Geometry check sheet. Reference: the model listing, model coordinates, mm. A direction names the side the tool comes from. Round coordinates to 2 decimals unless told otherwise and drop trailing zeros. Order: outer loops, then holes, each group sorted by start corner. A loop starts at its lowest first (then second) coordinate and runs counter-clockwise, first axis right, second up.
Autodesk Inventor part; units mm, degrees
ref_plane "Work Plane1" through (0, 0, 0) normal (0, 0, 1) x (1, 0, 0)
ref_plane "Work Plane2" through (0.04, -9.12, 0) normal (1, 0, 0) x (0, 0, -1)
ref_plane "YZ Plane" through (0, 0, 0) normal (1, 0, 0) x (0, 1, 0)
ref_plane "Work Plane1" through (0, 0, 0) normal (0, 0, 1) x (1, 0, 0)
sketch "Sketch1" plane through (0, 0, 0) normal (0, 0, 1) x (1, 0, 0)
  circle A0 centre (2.54, -6.27) radius 0.302
  circle A1 centre (-2.46, -6.27) radius 0.302
  line L0 (2.54, -6.27) -> (-2.46, -6.27)
  line L1 (2.89, -9.37) -> (-2.81, -9.37)
  line L2 (-3.06, -9.12) -> (-3.06, -3.42)
  line L3 (-2.81, -3.17) -> (2.89, -3.17)
  line L4 (3.14, -3.42) -> (3.14, -9.12)
  line L5 (3.14, -9.37) -> (-3.06, -3.17) construction
  line L6 (-3.06, -9.37) -> (3.14, -3.17) construction
  arc A2 (2.89, -9.37) -> (3.14, -9.12) centre (2.89, -9.12) ccw
  arc A3 (-3.06, -9.12) -> (-2.81, -9.37) centre (-2.81, -9.12) ccw
  arc A4 (-2.81, -3.17) -> (-3.06, -3.42) centre (-2.81, -3.42) ccw
  arc A5 (3.14, -3.42) -> (2.89, -3.17) centre (2.89, -3.42) ccw
  point P0 (0, 0)
  point P1 (0.04, -6.27)
  dimension "d0" = 6.2
  dimension "d1" = 6.2
  dimension "d2" = 0.25
extrude "Extrusion1" add sketch "Sketch1" along normal blind 3.4 contours A0 | A1 | L1 A3 L2 A4 L3 A5 L4 A2
sketch "Sketch2" plane through (0, 0, 3.4) normal (0, 0, 1) x (1, 0, 0)
  arc A0 (2.89, -9.37) -> (3.14, -9.12) centre (2.89, -9.12) ccw
  line L0 (3.14, -9.12) -> (3.14, -3.42)
  arc A1 (3.14, -3.42) -> (2.89, -3.17) centre (2.89, -3.42) ccw
  line L1 (2.89, -3.17) -> (-2.81, -3.17)
  arc A2 (-2.81, -3.17) -> (-3.06, -3.42) centre (-2.81, -3.42) ccw
  line L2 (-3.06, -3.42) -> (-3.06, -9.12)
  arc A3 (-3.06, -9.12) -> (-2.81, -9.37) centre (-2.81, -9.12) ccw
  line L3 (-2.81, -9.37) -> (2.89, -9.37)
  line L4 (-1.885, -4.345) -> (1.965, -8.195) construction
  line L5 (1.965, -4.345) -> (-1.885, -8.195) construction
  circle A4 centre (1.965, -4.345) radius 0.45
  circle A5 centre (1.965, -8.195) radius 0.45
  circle A6 centre (-1.885, -8.195) radius 0.45
  circle A7 centre (-1.885, -4.345) radius 0.45
  point P0 (0, 0)
  point P1 (0.04, -6.27)
  dimension "d5" = 3.85
  dimension "d6" = 3.85
  dimension "d7" = 0.9
  dimension "d8" = 0.9
  dimension "d9" = 0.9
  dimension "d10" = 0.9
extrude "Extrusion2" add sketch "Sketch2" along normal blind 0.4 contours A4 | A5 | A6 | A7
fillet "Fillet1" radius 0.1 4 edges at (1.515, -4.345, 3.8) (1.515, -8.195, 3.8) (-2.335, -8.195, 3.8) (-2.335, -4.345, 3.8)
sketch "Sketch3" plane through (0, 0, 3.4) normal (0, 0, 1) x (1, 0, 0)
  circle A0 centre (-1.885, -8.195) radius 0.45
  circle A1 centre (1.965, -8.195) radius 0.45
  circle A2 centre (-1.885, -4.345) radius 0.45
  circle A3 centre (1.965, -4.345) radius 0.45
  arc A4 (2.89, -9.37) -> (3.14, -9.12) centre (2.89, -9.12) ccw
  line L0 (3.14, -9.12) -> (3.14, -3.42)
  arc A5 (3.14, -3.42) -> (2.89, -3.17) centre (2.89, -3.42) ccw
  line L1 (2.89, -3.17) -> (-2.81, -3.17)
  arc A6 (-2.81, -3.17) -> (-3.06, -3.42) centre (-2.81, -3.42) ccw
  line L2 (-3.06, -3.42) -> (-3.06, -9.12)
  arc A7 (-3.06, -9.12) -> (-2.81, -9.37) centre (-2.81, -9.12) ccw
  line L3 (-2.81, -9.37) -> (2.89, -9.37)
  circle A8 centre (0.04, -6.27) radius 1.7
  point P0 (0, 0)
  dimension "d14" = 3.4
extrude "Extrusion3" add sketch "Sketch3" along normal blind 1.48 contours A8
fillet "Fillet2" radius 0.1 1 edges at (-1.66, -6.27, 4.88)
sketch "Sketch4" plane through (0, 0, 0) normal (0, 0, -1) x (-1, 0, 0)
  circle A0 centre (2.46, -6.27) radius 0.302
  circle A1 centre (-2.54, -6.27) radius 0.302
  point P0 (0, 0)
extrude "Extrusion4" add sketch "Sketch4" along normal blind 1.48
ref_plane "Work Plane2" through (0.04, -9.12, 0) normal (1, 0, 0) x (0, 0, -1)
properties part number "Button"
(1) Sectioned sample at A-A, the plane x = -2.46. Record the cut outline in (y, z).
Returned:
outline: (-9.37, 0) - (-6.57, 0) - (-6.57, -1.48) - (-5.97, -1.48) - (-5.97, 0) - (-3.17, 0) - (-3.17, 3.4) - (-9.37, 3.4) - close
(2) Sectioned sample at B-B, the plane y = -6.27. Record the cut outline in (x, z), and give its area (3 significant figures).
Returned:
outline: (-3.06, 0) - (-2.76, 0) - (-2.76, -1.48) - (-2.16, -1.48) - (-2.16, 0) - (2.24, 0) - (2.24, -1.48) - (2.84, -1.48) - (2.84, 0) - (3.14, 0) - (3.14, 3.4) - (1.74, 3.4) - (1.74, 4.78) arc R0.1 ccw to (1.64, 4.88) - (-1.56, 4.88) arc R0.1 ccw to (-1.66, 4.78) - (-1.66, 3.4) - (-3.06, 3.4) - close
area: 27.9 mm2
(3) Set-up check for faces 5 (the flat face through (-3.06, -6, 2)), 6 (the cylindrical face through (-0.181, -7.956, 4.08)): record each of +Z, -Z, +X, -X, +Y, -Y from which the full face is reachable in a straight line by a thin tool's end or side.
Returned:
face 5: +Z, -Z, -X, +Y, -Y
face 6: +Z
(4) Sectioned sample at C-C, the plane x = 0.04. Record the cut outline in (y, z), and give its area (3 significant figures).
Returned:
outline: (-9.37, 0) - (-3.17, 0) - (-3.17, 3.4) - (-4.57, 3.4) - (-4.57, 4.78) arc R0.1 ccw to (-4.67, 4.88) - (-7.87, 4.88) arc R0.1 ccw to (-7.97, 4.78) - (-7.97, 3.4) - (-9.37, 3.4) - close
area: 26.1 mm2
(5) Material ranges on line 1 (Z direction, x = 2.75, y = -3.5); line 2 (Y direction, x = -1.5, z = 3.5); line 3 (Z direction, x = -0.75, y = -6.5), recorded low to high.
Returned:
line 1: z = 0 to 3.4
line 2: y = -8.43 to -7.96, -6.99 to -5.55, -4.58 to -4.11
line 3: z = 0 to 4.88
(6) Depth check by flat-ended pin: P1, Ø1.9, axis at x = -1, y = -5.5, coming from the -Z side; P2, Ø0.8, axis at x = -2, y = -8, coming from the +Z side; P3, Ø1.5, axis at x = 2, z = -0.5, coming from the -Y side. Enter the tip coordinate at first touch or a pass-through.
Returned:
P1: stops at z = 0
P2: stops at z = 3.8
P3: stops at y = -9.37
(7) Draft check along Y on faces 1 (the flat face through (0, -3.17, 2)), 2 (the cylindrical face through (-1.94, -4.79, 3.55)), 3 (the flat face through (1.4, -4.8, 3.4)), 4 (the flat face through (0, -9.37, 2)). Enter one of: released by +Y, released by -Y, zero draft, split by the parting line, or undercut.
Returned:
face 1: released by +Y
face 2: undercut
face 3: undercut
face 4: released by -Y
